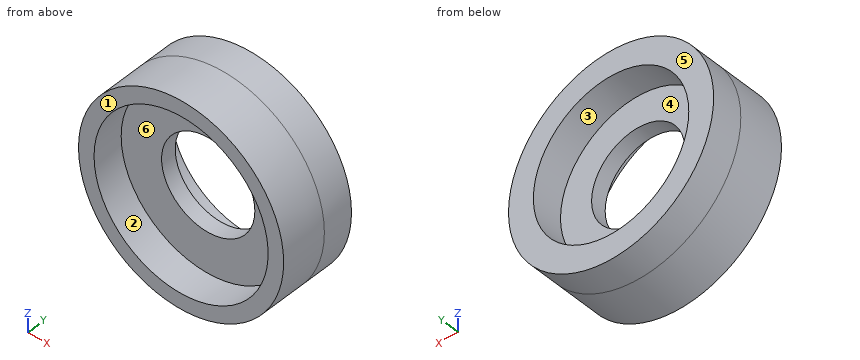
Autodesk Inventor part; units mm, degrees
ref_plane "YZ Plane" through (0, 0, 0) normal (1, 0, 0) x (0, 1, 0)
ref_plane "XZ Plane" through (0, 0, 0) normal (0, 1, 0) x (-1, 0, 0)
ref_plane "XY Plane" through (0, 0, 0) normal (0, 0, 1) x (1, 0, 0)
sketch "Sketch1" plane through (0, 0, 0) normal (0, 1, 0) x (-1, 0, 0)
  circle A0 centre (0, 0) radius 28
  circle A1 centre (0, 0) radius 33
  dimension "d0" = 56
  dimension "d1" = 66
extrude "Extrusion1" add sketch "Sketch1" along normal blind 10
sketch "Sketch2" plane through (0, 10, 0) normal (0, 1, 0) x (1, 0, 0)
  circle A0 centre (0, 0) radius 15
  circle A1 centre (0, 0) radius 33
  dimension "d4" = 30
extrude "Extrusion2" add sketch "Sketch2" along normal blind 5
sketch "Sketch3" plane through (0, 15, 0) normal (0, 1, 0) x (1, 0, 0)
  circle A0 centre (0, 0) radius 25
  circle A1 centre (0, 0) radius 33
  dimension "d7" = 66
  dimension "d8" = 50
extrude "Extrusion3" add sketch "Sketch3" along normal blind 10
properties part number "bigbearingcup" material "Steel"
Work out the finished part from the listing and answer in its coordinate system (mm). Face numbers are marked on the shaded views. A direction names the side the tool comes from. Coordinates: 2 decimals unless noted, no trailing zeros. Write each loop counter-clockwise with the first axis right and the second up, starting at its lowest first coordinate (ties: lowest second). Pieces come first, ordered by that corner, then holes. Notation, with made-up numbers: (45, 42.25) - (103, 42.25) arc R15 cw to (103, 60.25) - close; hole circle Ø6 at (78, 39). An arc over 180 degrees is marked (long way). Answer as a JSON object with one key per item and string values.
Q1. Consider L1, parallel to X at y = 18.5, z = 0; L2, parallel to Z at x = 0, y = 3; L3, parallel to X at y = 12.15, z = 0. Determine where each line is inside the solid, lowest interval first. Write a range as from..to.
Results list:
{"L1": "x = -33..-25, 25..33", "L2": "z = -33..-28, 28..33", "L3": "x = -33..-15, 15..33"}
Q2. Find section D-D (z = -18.5). Write down the section's boundary in (x, y), plus the area to 3 significant figures.
Results list:
{"outline": "(-27.33, 0) - (-21.02, 0) - (-21.02, 10) - (21.02, 10) - (21.02, 0) - (27.33, 0) - (27.33, 25) - (16.82, 25) - (16.82, 15) - (-16.82, 15) - (-16.82, 25) - (-27.33, 25) - close", "area": "610 mm^2"}
Q3. Find section C-C (y = 5.75). Write down the section's boundary in (x, z), plus the area to 3 significant figures.
Results list:
{"outline": "circle Ø66 at (0, 0); hole circle Ø56 at (0, 0)", "area": "958 mm^2"}
Q4. Which of the six approach directions +Z, -Z, +X, -X, +Y, -Y give full straight-line access (tool end or side, diameter ignored) to the marked faces 1, 2 and 3?
Results list:
{"face 1": "+Z, -Z, +X, -X, -Y", "face 2": "-Y", "face 3": "+Y"}
Q5. Find section B-B (z = -5). Write down the section's boundary in (x, y), plus the area to 3 significant figures.
Results list:
{"outline": "(-32.62, 0) - (-27.55, 0) - (-27.55, 10) - (-14.14, 10) - (-14.14, 15) - (-24.49, 15) - (-24.49, 25) - (-32.62, 25) - close; (14.14, 10) - (27.55, 10) - (27.55, 0) - (32.62, 0) - (32.62, 25) - (24.49, 25) - (24.49, 15) - (14.14, 15) - close", "area": "449 mm^2"}
Q6. For a pull along Z with two mould halves and no side action, classify the marked faces 4, 5 and 6 as pulls with the +Z half, pulls with the -Z half, needs draft (parallel to the pull), parting line crosses it, or undercut.
Results list:
{"face 4": "undercut", "face 5": "needs draft", "face 6": "undercut"}
Q7. Given pin 1 Ø10 at (x, y) = (5, 18) entering from +Z; pin 2 Ø5 at (x, z) = (15.5, -7.5) entering from +Y; pin 3 Ø12 at (y, z) = (17.5, 20.5) entering from +X, each flat-ended and moving along its own axis, determine where each tip first touches the part or whether it passes through.
Results list:
{"pin 1": "stops at z = 33", "pin 2": "stops at y = 15", "pin 3": "stops at x = 29.64"}
